from build123d import *


with BuildPart() as part:
    # Sketch1 → Revolve2 (revolve)
    with BuildSketch(Plane.XY, mode=Mode.PRIVATE) as revolve2_sk:
        Polygon((8, 5), (8, 0), (12, 0), (12, 3), (10, 5), align=None)
    revolve2 = revolve(revolve2_sk.sketch.rotate(Axis((0, 0, 0), (0, 1, 0)), 90), axis=Axis((0, 0, 0), (0, 1, 0)))

    # Mirror1: Revolve2 across plane
    add(revolve2.mirror(Plane(origin=(0, 0, 0), x_dir=(0, 0, 1), z_dir=(0, -1, 0))))


solid = part.part
Check sheet for the modelled part. Datum: model origin and axes. Units: mm. Round coordinates to 2 decimals unless told otherwise and drop trailing zeros. Order: outer loops, then holes, each group sorted by start corner. A loop starts at its lowest first (then second) coordinate and runs counter-clockwise, first axis right, second up.
(1) Go/stop test with flat-tipped pins: P1, Ø6, axis at x = -9.5, y = 2, coming from the -Z side; P2, Ø1.5, axis at x = -6.5, y = -2.5, coming from the +Z side; P3, Ø3, axis at x = -9, z = -9, coming from the -Y side. Record where each tip stops, or that it passes through.
(2) Scan lines: probe 1 along X at (y, z) = (2.5, 0); probe 2 along X at (y, z) = (2.25, -2.25); probe 3 along Z at (x, y) = (-0.5, -2.5). Record each from-to range of solid material in increasing order.
(3) Cross-section at C-C, the plane y = 2. Enter the section's corners in (x, z), and give its area (3 significant figures).
(4) Draft check along Y on faces 1 (the flat face through (-8.2, 5, 0)), 2 (the flat face through (-8.2, -5, 0)). Enter one of: pulls with the +Y half, pulls with the -Y half, needs draft (parallel to the pull), parting line crosses it, or undercut.
(5) Cross-section at D-D, the plane y = 3.75. Enter the section's corners in (x, z), and give its area (3 significant figures).
(6) Cross-section at A-A, the plane x = 0. Enter the section's corners in (y, z).
(7) Cross-section at B-B, the plane z = 0. Enter the section's corners in (x, y), and give its area (3 significant figures).
Check sheet entries:
1. P1: stops at z = -10.09
1. P2: stops at z = 10.53
1. P3: stops at y = -3.77
2. probe 1: x = -12 to -8, 8 to 12
2. probe 2: x = -11.79 to -7.68, 7.68 to 11.79
2. probe 3: z = -11.99 to -7.98, 7.98 to 11.99
3. outline: circle Ø24 at (0, 0); hole circle Ø16 at (0, 0)
3. area: 251 mm2
4. face 1: pulls with the +Y half
4. face 2: pulls with the -Y half
5. outline: circle Ø22.5 at (0, 0); hole circle Ø16 at (0, 0)
5. area: 197 mm2
6. outline: (-5, -10) - (-3, -12) - (3, -12) - (5, -10) - (5, -8) - (-5, -8) - close; (-5, 8) - (5, 8) - (5, 10) - (3, 12) - (-3, 12) - (-5, 10) - close
7. outline: (-12, -3) - (-10, -5) - (-8, -5) - (-8, 5) - (-10, 5) - (-12, 3) - close; (8, -5) - (10, -5) - (12, -3) - (12, 3) - (10, 5) - (8, 5) - close
7. area: 72.0 mm2
